Design review of the part built by this model. Coordinates are the model's own, in mm. Give positions to 0.01 mm unless a question says otherwise; leave off trailing zeros. Loops run counter-clockwise (first coordinate to the right, second up) from the corner with the lowest first, then second, coordinate; pieces in that order, holes last.
from build123d import *

# Parameters (mm, degrees)
SKETCH1_R           = 115
SKETCH1_R_2         = 1.75
BOSS_EXTRUDE1_DEPTH = 0.1
BOSS_EXTRUDE2_DEPTH = 2


with BuildPart() as part:
    # Sketch1 → Boss-Extrude1 (new body)
    with BuildSketch(Plane.XY):
        Circle(SKETCH1_R)
        Circle(SKETCH1_R_2, mode=Mode.SUBTRACT)
    extrude(amount=BOSS_EXTRUDE1_DEPTH)

    # Sketch2 → Boss-Extrude2 (add)
    with BuildSketch(Plane.XY.offset(0.1)):
        Polygon((2.75, 102), (1, 103.75), (-1, 103.75), (-2.75, 102), align=None)
        Polygon((-31.536422151, 98.845923426), (-32.692853006, 96.657849461), (-34.314006465, 101.913499892), (-32.383843277, 101.593195243), align=None)
        Polygon((-61.876050067, 88.980307108), (-62.829062871, 87.271538079), (-65.927323191, 91.815851338), (-63.495595234, 91.355743585), align=None)
        Polygon((-86.355262623, 70.145071939), (-87.602242226, 68.581408974), (-90.061554474, 68.304311033), (-86.632360564, 72.604384187), align=None)
        Polygon((-104.18404578, 43.843438562), (-103.194363512, 41.575062709), (-100.518101485, 40.524707264), (-99.064240162, 41.834062928), align=None)
        Polygon((-106.252124781, 8.965300026), (-106.99390044, 10.775795503), (-101.509279555, 10.364779988), (-103.385163864, 8.750451007), align=None)
        Polygon((-105.416683128, -21.239948642), (-105.880333417, -23.140778305), (-105.435291549, -25.09063413), (-104.192817991, -26.602052159), (-103.729167702, -24.701222495), (-104.17420957, -22.751366671), align=None)
        Polygon((-86.959591186, -53.38156986), (-89.709591186, -48.61843014), (-90.350135643, -51.008974596), (-89.350135643, -52.741025404), align=None)
        Polygon((-69.834869672, -76.73430444), (-67.361726605, -76.641765956), (-71.102676663, -80.673551251), (-71.790366293, -78.841828572), align=None)
        Polygon((-46.121181359, -98.076384798), (-44.164837568, -98.047333582), (-46.551198134, -103.002662356), (-47.368597109, -100.666670293), align=None)
        Polygon((-17.569782938, -109.858387151), (-15.592121286, -110.156471684), (-14.122491306, -112.147749595), (-19.56106085, -111.328017131), align=None)
        Polygon((14.122491306, -112.147749595), (15.592121286, -110.156471684), (15.163624771, -107.313583058), (13.302758842, -106.709180051), align=None)
        Polygon((45.361884816, -96.499689279), (44.164837568, -98.047333582), (41.778477003, -93.092004809), (44.114469066, -93.909403784), align=None)
        Polygon((71.102676663, -80.673551251), (72.980668584, -80.124669347), (74.446772328, -78.764323872), (75.134461958, -76.932601193), (73.256470037, -77.481483096), (71.790366293, -78.841828572), align=None)
        Polygon((89.709591186, -48.61843014), (86.959591186, -53.38156986), (89.350135643, -52.741025404), (90.350135643, -51.008974596), align=None)
        Polygon((101.371291823, -22.111618986), (100.054579611, -20.016083505), (105.416683128, -21.239948642), (104.17420957, -22.751366671), align=None)
        Polygon((107.997231426, 9.09607769), (106.99390044, 10.775795503), (112.478521324, 11.186811018), (110.864192343, 9.310926709), align=None)
        Polygon((103.925045561, 39.713315212), (103.194363512, 41.575062709), (104.18404578, 43.843438562), (106.193421414, 38.723632945), align=None)
        Polygon((90.061554474, 68.304311033), (87.602242226, 68.581408974), (85.354476714, 66.788875794), (85.76148132, 64.875117123), align=None)
        Polygon((60.890239965, 87.534389253), (62.829062871, 87.271538079), (59.730802552, 82.727224821), (59.270694798, 85.158952777), align=None)
        Polygon((34.314006465, 101.913499892), (32.899664833, 103.265447653), (30.988519221, 103.854958001), (29.058356033, 103.534653352), (30.472697666, 102.182705591), (32.383843277, 101.593195243), align=None)
    extrude(amount=BOSS_EXTRUDE2_DEPTH)


solid = part.part
Q1. Take a section at B-B (x = 5.5). Give the boundary of the cut face in (y, z), plus the area to 3 significant figures.
Results:
outline: (-114.87, 0) - (114.87, 0) - (114.87, 0.1) - (-114.87, 0.1) - close
area: 23.0 mm2
Q2. Take a section at C-C (y = -34). Give the boundary of the cut face in (x, z), plus the area to 3 significant figures.
Results:
outline: (-109.86, 0) - (109.86, 0) - (109.86, 0.1) - (-109.86, 0.1) - close
area: 22.0 mm2
Q3. Take a section at A-A (z = 1.15). Give the number of separate pieces and of enclosed holes in the cut face, plus the area to 3 significant figures.
Results:
separate pieces: 21
enclosed holes: 0
area: 147 mm2
Q4. Wall thickness on line 1 (Y direction, x = 0, z = 0.05); line 2 (Y direction, x = -1, z = 0.8); line 3 (X direction, y = -25.5, z = 1.75): over which ranges is each line inside the solid? List them lowest first.
Results:
line 1: y = -115 to -1.75, 1.75 to 115
line 2: y = 102 to 103.75
line 3: x = -105.1 to -103.92
Q5. Insertion check: pin 1 (1 mm diameter, centred on y = -83, z = 0.5, fed in from +X); pin 2 (1.5 mm diameter, centred on x = 51, y = 56.5, fed in from +Z); pin 3 (0.6 mm diameter, centred on x = 1, z = 1, fed in from -Y); pin 4 (2 mm diameter, centred on x = 0, y = 0, fed in from +Z). Each pin has a flat end and moves straight along its axis. Give the tip position at first contact, or say it passes through.
Results:
pin 1: stops at x = 79.91
pin 2: stops at z = 0.1
pin 3: stops at y = 102
pin 4: passes through
